from build123d import *

# Parameters (mm, degrees)
EXTRUDE_THIN1_START            = -40
SKETCH1_W                      = 38.1
SKETCH1_H                      = 76.2
SKETCH1_W_2                    = 31.75
SKETCH1_H_2                    = 69.85
EXTRUDE_THIN1_DEPTH            = 170
M8_CLEARANCE_HOLE2_D           = 9
M8_CLEARANCE_HOLE3_D           = 9
F_12_0_12_DIAMETER_HOLE1_D     = 12
F_12_0_12_DIAMETER_HOLE1_DEPTH = 3.175


with BuildPart() as part:
    # Sketch1 → Extrude-Thin1 (new body)
    with BuildSketch(Plane(origin=(0, 0, 0), x_dir=(0, 0, -1), z_dir=(1, 0, 0)).offset(EXTRUDE_THIN1_START)):
        Rectangle(SKETCH1_W, SKETCH1_H)
        Rectangle(SKETCH1_W_2, SKETCH1_H_2, mode=Mode.SUBTRACT)
    extrude(amount=EXTRUDE_THIN1_DEPTH)

    # M8 Clearance Hole2 (through all)
    with Locations(Plane(origin=(0, 0, -19.05), x_dir=(-1, 0, 0), z_dir=(0, 0, -1))):
        with Locations((20, -18.1), (-20, -18.1), (-60, -18.1)):
            Hole(M8_CLEARANCE_HOLE2_D / 2)

    # M8 Clearance Hole3 (through all)
    with Locations(Plane(origin=(0, -38.1, 0), x_dir=(-1, 0, 0), z_dir=(0, -1, 0))):
        with Locations((-20, 0), (20, 0)):
            Hole(M8_CLEARANCE_HOLE3_D / 2)

    # Ø12.0 (12) Diameter Hole1
    with Locations(Plane(origin=(0, 0, -19.05), x_dir=(-1, 0, 0), z_dir=(0, 0, -1))):
        with Locations((-118, -18.1), (-82, -18.1)):
            Hole(F_12_0_12_DIAMETER_HOLE1_D / 2, depth=F_12_0_12_DIAMETER_HOLE1_DEPTH)


solid = part.part
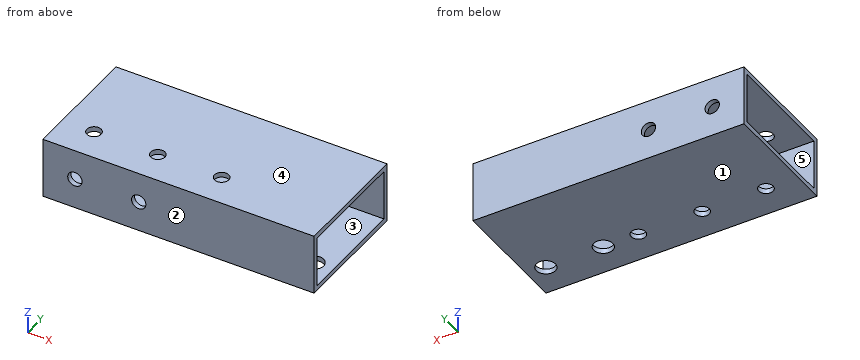
Work out the finished part from the listing and answer in its coordinate system (mm). Face numbers are marked on the shaded views. A direction names the side the tool comes from. Coordinates: 2 decimals unless noted, no trailing zeros. Loops run counter-clockwise (first coordinate to the right, second up) from the corner with the lowest first, then second, coordinate; pieces in that order, holes last. Notation, with made-up numbers: (-16.5, 89) -> (18.5, 89) arc R24 cw to (18.5, 112) -> close; hole circle Ø11 at (74.5, 34.5). An arc over 180 degrees is marked (long way). Answer as CSV lines item,"result".
1) The part is cut by section A-A (y = 8). Give the vertices of the cut face in (x, z) (3 decimals).
A:
outline,"(-40, -19.05) -> (130, -19.05) -> (130, -15.875) -> (-40, -15.875) -> close; (-40, 15.875) -> (130, 15.875) -> (130, 19.05) -> (-40, 19.05) -> close"
2) The part is cut by section B-B (z = -14). Give the vertices of the cut face in (x, y) (3 decimals), and give its area (3 significant figures).
A:
outline,"(-40, -38.1) -> (130, -38.1) -> (130, -34.925) -> (-40, -34.925) -> close; (-40, 34.925) -> (130, 34.925) -> (130, 38.1) -> (-40, 38.1) -> close"
area,"1,080 mm²"
3) The part is cut by section C-C (x = -20). Give the vertices of the cut face in (y, z) (3 decimals).
A:
outline,"(-38.1, -19.05) -> (-22.6, -19.05) -> (-22.6, -15.875) -> (-34.925, -15.875) -> (-34.925, -4.5) -> (-38.1, -4.5) -> close; (-38.1, 4.5) -> (-34.925, 4.5) -> (-34.925, 15.875) -> (-22.6, 15.875) -> (-22.6, 19.05) -> (-38.1, 19.05) -> close; (-13.6, -19.05) -> (38.1, -19.05) -> (38.1, -4.5) -> (34.925, -4.5) -> (34.925, -15.875) -> (-13.6, -15.875) -> close; (-13.6, 15.875) -> (34.925, 15.875) -> (34.925, 4.5) -> (38.1, 4.5) -> (38.1, 19.05) -> (-13.6, 19.05) -> close"
4) Straight lines are drawn through the part: probe 1 along X at (y, z) = (-18, 17); probe 2 along Z at (x, y) = (49, 8) (3 decimals); probe 3 along Z at (x, y) = (20, 37). For each, find the intervals that lie inside material, in ascending order.
A:
probe 1,"x = -40 to -24.5, -15.5 to 15.5, 24.5 to 55.5, 64.5 to 130"
probe 2,"z = -19.05 to -15.875, 15.875 to 19.05"
probe 3,"z = -19.05 to -4.5, 4.5 to 19.05"
5) Flat-ended cylindrical pins translate along their axes: pin 1 (9.5 mm diameter, centred on x = 82, y = -18.1, fed in from -Z) (3 decimals); pin 2 (8 mm diameter, centred on x = 20, y = -18.1, fed in from +Z). Find the tip coordinate at first contact, or state that the pin passes through.
A:
pin 1,"stops at z = 15.875"
pin 2,"passes through"
6) The part is cut by section D-D (z = 0). Give the vertices of the cut face in (x, y) (3 decimals), and give its area (3 significant figures).
A:
outline,"(-40, -38.1) -> (-24.5, -38.1) -> (-24.5, -34.925) -> (-40, -34.925) -> close; (-40, 34.925) -> (-24.5, 34.925) -> (-24.5, 38.1) -> (-40, 38.1) -> close; (-15.5, -38.1) -> (15.5, -38.1) -> (15.5, -34.925) -> (-15.5, -34.925) -> close; (-15.5, 34.925) -> (15.5, 34.925) -> (15.5, 38.1) -> (-15.5, 38.1) -> close; (24.5, -38.1) -> (130, -38.1) -> (130, -34.925) -> (24.5, -34.925) -> close; (24.5, 34.925) -> (130, 34.925) -> (130, 38.1) -> (24.5, 38.1) -> close"
area,"965 mm²"
7) For a pull along Y with two mould halves and no side action, classify the marked faces 1, 2 and 3 as released by +Y, released by -Y, zero draft, split by the parting line, or undercut.
A:
face 1,"zero draft"
face 2,"released by -Y"
face 3,"undercut"
8) For the marked faces 4 and 5, determine the directions among +Z, -Z, +X, -X, +Y, -Y from which every point of the face is accessible in a straight line to the end or side of a thin tool.
A:
face 4,"+Z, +X, -X, +Y, -Y"
face 5,"+X, -X"
